The listing builds one solid part. Answer for the finished solid, in the listing's coordinates (mm). Face numbers are marked on the shaded views. A direction names the side the tool comes from. Round coordinates to 2 decimals unless told otherwise and drop trailing zeros. Loops run counter-clockwise (first coordinate to the right, second up) from the corner with the lowest first, then second, coordinate; pieces in that order, holes last. Notation, with made-up numbers: M 17,6 L 36,6 A13 ccw 36,22 Z; hole C -25.5,24.25 d9. An arc over 180 degrees is marked long. Put each result on its own line as item: value. Start each with the question number.
(1) Section C-C, the plane y = 24.5 is taken. Determine the outline of the cut face in (x, z) (1 decimal).
(2) Which of the six approach directions +Z, -Z, +X, -X, +Y, -Y give full straight-line access (tool end or side, diameter ignored) to the marked faces 1, 2, 3 and 4?
(3) Section B-B, the plane x = -2.5 is taken. Determine the outline of the cut face in (y, z) (1 decimal).
(4) Section D-D, the plane z = 4.5 is taken. Determine the outline of the cut face in (x, y) (3 decimals).
(5) Section A-A, the plane z = 0 is taken. Determine the outline of the cut face in (x, y).
(6) Straight lines are drawn through the part: line 1 (Y direction, x = 0.5, z = 16); line 2 (Y direction, x = -5.25, z = 8.5); line 3 (X direction, y = 3.25, z = 0). For each, find the intervals that lie inside material, in ascending order.
(7) Flat-ended cylindrical pins translate along their axes: P1, Ø1, axis at x = 9.5, y = 8.5, coming from the +Z side; P2, Ø8.5, axis at x = 3, z = 14.5, coming from the +Y side; P3, Ø6, axis at x = 7.5, z = -2, coming from the +Y side; P4, Ø5, axis at y = 15.5, z = -8, coming from the +X side. Find the tip coordinate at first contact, or state that the pin passes through.
```python
from build123d import *
from build123d.topology import SkipClean

# Parameters (mm, degrees)
SKETCH1_R           = 12.0015
BOSS_EXTRUDE1_DEPTH = 7.62
SKETCH2_R           = 12.7
BOSS_EXTRUDE2_DEPTH = 1.27
BOSS_EXTRUDE3_START = -1.27
BOSS_EXTRUDE3_DEPTH = 1.27
SKETCH4_R           = 5.9944
BOSS_EXTRUDE4_DEPTH = 2.6162
SKETCH5_R           = 4.0005
BOSS_EXTRUDE5_DEPTH = 6.5024
SKETCH6_R           = 3.4925
BOSS_EXTRUDE6_DEPTH = 8.509
BOSS_EXTRUDE7_DEPTH = 0.635
BOSS_EXTRUDE8_DEPTH = 0.635


with BuildPart() as part:
    # Sketch1 → Boss-Extrude1 (new body)
    with BuildSketch(Plane(origin=(0, 0, 0), x_dir=(1, 0, 0), z_dir=(0, 1, 0))):
        with Locations(Location((0, 0, 0), (0, 0, 90))):
            Circle(SKETCH1_R)
    extrude(amount=BOSS_EXTRUDE1_DEPTH)

    # Sketch2 → Boss-Extrude2 (add)
    with BuildSketch(Plane(origin=(0, 7.62, 0), x_dir=(1, 0, 0), z_dir=(0, 1, 0))):
        with Locations(Location((0, 0, 0), (0, 0, 270))):
            Circle(SKETCH2_R)
    extrude(amount=BOSS_EXTRUDE2_DEPTH)

    # Sketch3 → Boss-Extrude3 (add)
    with BuildSketch(Plane(origin=(0, 8.89, 0), x_dir=(1, 0, 0), z_dir=(0, 1, 0)).offset(BOSS_EXTRUDE3_START)):
        with BuildLine():
            ThreePointArc((9.9949, -7.835303057), (0, -12.7), (-9.9949, -7.835303057))
            Line((-9.9949, -7.835303057), (-9.9949, -11.612260807))
            Line((-9.9949, -11.612260807), (-8.7249, -11.612260807))
            Line((-8.7249, -11.612260807), (-8.7249, -12.882260807))
            Line((-8.7249, -12.882260807), (-9.9949, -12.882260807))
            Line((-9.9949, -12.882260807), (-9.9949, -15.422260807))
            ThreePointArc((-9.9949, -15.422260807), (0, -17.6022), (9.9949, -15.422260807))
            Line((9.9949, -15.422260807), (9.9949, -12.882260807))
            Line((9.9949, -12.882260807), (8.7249, -12.882260807))
            Line((8.7249, -12.882260807), (8.7249, -11.612260807))
            Line((8.7249, -11.612260807), (9.9949, -11.612260807))
            Line((9.9949, -11.612260807), (9.9949, -7.835303057))
        make_face()
    extrude(amount=BOSS_EXTRUDE3_DEPTH)

    # Sketch4 → Boss-Extrude4 (add)
    with BuildSketch(Plane(origin=(0, 8.89, 0), x_dir=(1, 0, 0), z_dir=(0, 1, 0))):
        with Locations(Location((0, 0, 0), (0, 0, 270))):
            Circle(SKETCH4_R)
    extrude(amount=BOSS_EXTRUDE4_DEPTH)

    # Sketch5 → Boss-Extrude5 (add)
    with BuildSketch(Plane(origin=(0, 11.5062, 0), x_dir=(1, 0, 0), z_dir=(0, 1, 0))):
        with Locations(Location((0, 0, 0), (0, 0, 270))):
            Circle(SKETCH5_R)
    extrude(amount=BOSS_EXTRUDE5_DEPTH)

    # Sketch6 → Boss-Extrude6 (add)
    with BuildSketch(Plane(origin=(0, 18.0086, 0), x_dir=(1, 0, 0), z_dir=(0, 1, 0))):
        with Locations(Location((0, 0, 0), (0, 0, 270))):
            Circle(SKETCH6_R)
    extrude(amount=BOSS_EXTRUDE6_DEPTH)

    # Sketch7 → Boss-Extrude7 (add)
    with SkipClean():  # the faces are left unmerged after this step: merging them gives an invalid solid
        with BuildSketch(Plane(origin=(0, 8.89, 0), x_dir=(1, 0, 0), z_dir=(0, 1, 0))):
            with BuildLine():
                Line((-9.728764428, 8.163402643), (-3.11582165, 8.163402643))
                Line((-3.11582165, 8.163402643), (-1.905, 7.147402643))
                Line((-1.905, 7.147402643), (1.905, 7.147402643))
                Line((1.905, 7.147402643), (3.11582165, 8.163402643))
                Line((3.11582165, 8.163402643), (9.728764428, 8.163402643))
                ThreePointArc((9.728764428, 8.163402643), (12.7, 0), (9.728764428, -8.163402643))
                Line((9.728764428, -8.163402643), (3.11582165, -8.163402643))
                Line((3.11582165, -8.163402643), (1.905, -7.147402643))
                Line((1.905, -7.147402643), (-1.905, -7.147402643))
                Line((-1.905, -7.147402643), (-3.11582165, -8.163402643))
                Line((-3.11582165, -8.163402643), (-9.728764428, -8.163402643))
                ThreePointArc((-9.728764428, -8.163402643), (-12.7, 0), (-9.728764428, 8.163402643))
            make_face()
        extrude(amount=BOSS_EXTRUDE7_DEPTH)

    # Sketch8 → Boss-Extrude8 (add)
    with SkipClean():  # the faces are left unmerged after this step: merging them gives an invalid solid
        with BuildSketch(Plane(origin=(0, 9.525, 0), x_dir=(1, 0, 0), z_dir=(0, 1, 0))):
            with BuildLine():
                Line((-12.622931157, 1.397), (12.622931157, 1.397))
                ThreePointArc((12.622931157, 1.397), (12.7, 0), (12.622931157, -1.397))
                Line((12.622931157, -1.397), (-12.622931157, -1.397))
                ThreePointArc((-12.622931157, -1.397), (-12.7, 0), (-12.622931157, 1.397))
            make_face()
        extrude(amount=BOSS_EXTRUDE8_DEPTH)


solid = part.part
```
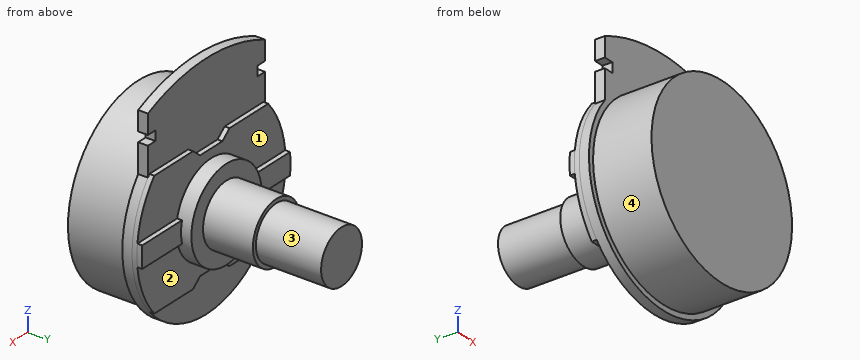
Recorded:
1. outline: C 0,0 d7
2. face 1: +Z, +Y
2. face 2: -Z, +Y
2. face 3: +Y
2. face 4: -Y
3. outline: M 0,-11.7 L 7.6,-11.7 L 7.6,-12.5 L 8.9,-12.5 L 8.9,-7.6 L 9.5,-7.6 L 9.5,-5.4 L 11.5,-5.4 L 11.5,-3.1 L 18,-3.1 L 18,-2.4 L 26.5,-2.4 L 26.5,2.4 L 18,2.4 L 18,3.1 L 11.5,3.1 L 11.5,5.4 L 9.5,5.4 L 9.5,7.6 L 8.9,7.6 L 8.9,17.5 L 7.6,17.5 L 7.6,11.7 L 0,11.7 Z
4. outline: M -11.876,7.62 L -11.126,7.62 L -11.126,0 L 11.126,0 L 11.126,7.62 L 11.876,7.62 L 11.876,9.525 L 3.96,9.525 L 3.96,11.506 L -3.96,11.506 L -3.96,9.525 L -11.876,9.525 Z
5. outline: M -12.7,7.62 L -12,7.62 L -12,0 L 12,0 L 12,7.62 L 12.7,7.62 L 12.7,10.16 L 5.99,10.16 L 5.99,11.51 L 4,11.51 L 4,18.01 L 3.49,18.01 L 3.49,26.52 L -3.49,26.52 L -3.49,18.01 L -4,18.01 L -4,11.51 L -5.99,11.51 L -5.99,10.16 L -12.7,10.16 Z
6. line 1: y = 7.62 to 8.89
6. line 2: y = 0 to 8.89
6. line 3: x = -12 to 12
7. P1: stops at z = 15.85
7. P2: stops at y = 8.89
7. P3: stops at y = 11.51
7. P4: passes through
